from build123d import *

# Parameters (mm, degrees)
EXTRUDE_1_DEPTH     = 4
CUT_EXTRUDE_1_DEPTH = 3
SKETCH_5_R          = 1.25
CUT_EXTRUDE_2_DEPTH = 12.4
SKETCH_13_W         = 36
SKETCH_13_H         = 45
EXTRUDE_2_DEPTH     = 37
SKETCH_14_W         = 13
SKETCH_14_H         = 24
CUT_EXTRUDE_3_DEPTH = 35
SKETCH_15_R         = 1.15
CUT_EXTRUDE_4_DEPTH = 31
SKETCH_16_W         = 10
SKETCH_16_H         = 8
CUT_EXTRUDE_5_DEPTH = 8
SKETCH_17_W         = 36
SKETCH_17_H         = 42.5
CUT_EXTRUDE_6_DEPTH = 18
SKETCH_23_R         = 1.15
CUT_EXTRUDE_7_DEPTH = 5
SKETCH_24_R         = 1.15
CUT_EXTRUDE_8_DEPTH = 5


with BuildPart() as part:
    # 草圖1 → 填料-伸長1 (new body)
    with BuildSketch(Plane.XY):
        with BuildLine():
            Line((7.5, 10), (7.5, 52))
            ThreePointArc((7.5, 52), (0, 59.5), (-7.5, 52))
            Line((-7.5, 52), (-7.5, 10))
            Line((-7.5, 10), (7.5, 10))
        make_face()
    extrude(amount=EXTRUDE_1_DEPTH)

    # 草圖3 → 除料-伸長1 (cut)
    with BuildSketch(Plane.XY):
        with BuildLine():
            ThreePointArc((-2.132795501, 52), (0, 54.132795501), (2.132795501, 52))
            Line((2.132795501, 52), (5, 34.5))
            Line((5, 34.5), (2.114741289, 16.658021353))
            ThreePointArc((2.114741289, 16.658021353), (-0.171540182, 14.864665347), (-2.142213835, 17))
            Line((-2.142213835, 17), (-5, 34.5))
            Line((-5, 34.5), (-2.132795501, 52))
        make_face()
    extrude(amount=CUT_EXTRUDE_1_DEPTH, mode=Mode.SUBTRACT)

    # 草圖5 → 除料-伸長2 (cut)
    with BuildSketch(Plane.XY):
        with Locations((0, 34.5)):
            Circle(SKETCH_5_R)
    extrude(amount=CUT_EXTRUDE_2_DEPTH, mode=Mode.SUBTRACT)

    # 草圖13 → 填料-伸長2 (add)
    with BuildSketch(Plane.XY.offset(4)):
        with Locations((0, -12.5)):
            Rectangle(SKETCH_13_W, SKETCH_13_H)
    extrude(amount=-EXTRUDE_2_DEPTH)

    # 草圖14 → 除料-伸長3 (cut)
    with BuildSketch(Plane(origin=(0, 0, 4), x_dir=(-1, 0, 0), z_dir=(0, 0, -1))):
        with Locations((0, -17)):
            Rectangle(SKETCH_14_W, SKETCH_14_H)
    extrude(amount=CUT_EXTRUDE_3_DEPTH, mode=Mode.SUBTRACT)

    # 草圖15 → 除料-伸長4 (cut)
    with BuildSketch(Plane.XY.offset(4)):
        with Locations((0, -1.85)):
            Circle(SKETCH_15_R)
        with Locations((0, -32.65)):
            Circle(SKETCH_15_R)
    extrude(amount=-CUT_EXTRUDE_4_DEPTH, mode=Mode.SUBTRACT)

    # 草圖16 → 除料-伸長5 (cut)
    with BuildSketch(Plane(origin=(0, -35, 0), x_dir=(-1, 0, 0), z_dir=(0, -1, 0))):
        with Locations((0, 25)):
            Rectangle(SKETCH_16_W, SKETCH_16_H)
    extrude(amount=-CUT_EXTRUDE_5_DEPTH, mode=Mode.SUBTRACT)

    # 草圖17 → 除料-伸長6 (cut)
    with BuildSketch(Plane.XY.offset(4)):
        with Locations((0, -13.75)):
            Rectangle(SKETCH_17_W, SKETCH_17_H)
    extrude(amount=-CUT_EXTRUDE_6_DEPTH, mode=Mode.SUBTRACT)

    # 草圖23 → 除料-伸長7 (cut)
    with BuildSketch(Plane.ZY.offset(18)):
        with Locations((-30, 7)):
            Circle(SKETCH_23_R)
        with Locations((-30, -32)):
            Circle(SKETCH_23_R)
    extrude(amount=-CUT_EXTRUDE_7_DEPTH, mode=Mode.SUBTRACT)

    # 草圖24 → 除料-伸長8 (cut)
    with BuildSketch(Plane(origin=(18, 0, 0), x_dir=(0, 0, -1), z_dir=(1, 0, 0))):
        with Locations((30, 7)):
            Circle(SKETCH_24_R)
        with Locations((30, -32)):
            Circle(SKETCH_24_R)
    extrude(amount=-CUT_EXTRUDE_8_DEPTH, mode=Mode.SUBTRACT)


solid = part.part
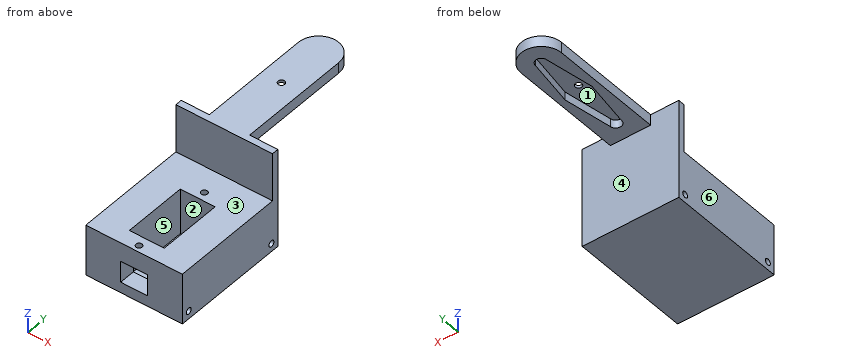
Can you work these out from the model? Positions are in its coordinate system, mm. Face numbers are marked on the shaded views. A direction names the side the tool comes from. Coordinates: 2 decimals unless noted, no trailing zeros. Loops run counter-clockwise (first coordinate to the right, second up) from the corner with the lowest first, then second, coordinate; pieces in that order, holes last. Notation, with made-up numbers: (40, -5) - (58, -5) arc R27 cw to (58, 11) - close; hole circle Ø3 at (72.25, 33). An arc over 180 degrees is marked (long way). Answer as a JSON object with one key per item and string values. Group by question number.
Item 1: On a 3-axis mill with a long thin cutter (end or side, diameter ignored), from which of +Z, -Z, +X, -X, +Y, -Y can I reach the whole of each face in a straight line? I mean the marked faces 1, 2 and 3. Say none if no direction works.
Item 2: If we section it at B-B (z = -25.5): List the corners of the cut face in (x, y) for me, plus the area to 3 significant figures.
Item 3: For pin 1 (5 mm diameter, centred on x = 12.5, z = -1.5, fed in from -Y); pin 2 (5 mm diameter, centred on x = 9, z = -18, fed in from +Y); pin 3 (8 mm diameter, centred on x = 9, y = 13, fed in from -Z); pin 4 (2.5 mm diameter, centred on x = 0, y = -2.5, fed in from +Z), each with a flat end and sliding along its axis, tell me the tip position at first contact or that it passes through.
Item 4: If we section it at D-D (z = -15): List the corners of the cut face in (x, y) for me, plus the area to 3 significant figures.
Item 5: If I drill on L1, parallel to Y at x = -16.05, z = -30; L2, parallel to X at y = -12.5, z = -28; L3, parallel to Y at x = 0, z = -16.25, over which ranges is the centre line in solid material (lowest first)? Write a range as from..to.
Item 6: If we mould it in two halves opening along Y, with no side actions, what happens to the marked faces 4, 5 and 6? For each: released by +Y, released by -Y, zero draft, split by the parting line, or undercut.
Item 7: If we section it at C-C (y = -21): List the corners of the cut face in (x, z) for me.
Item 8: If we section it at A-A (x = 0): State how many separate pieces and enclosed holes the cut face has, plus the area to 3 significant figures.
Returned:
{
 "1": {"face 1": "-Z", "face 2": "+Z", "face 3": "+Z, +X, -X, -Y"},
 "2": {"outline": "(-18, -35) - (-5, -35) - (-5, -29) - (-6.5, -29) - (-6.5, -5) - (6.5, -5) - (6.5, -29) - (5, -29) - (5, -35) - (18, -35) - (18, 10) - (-18, 10) - close; hole circle Ø2.3 at (0, -1.85)", "area": "1,240 mm²"},
 "3": {"pin 1": "stops at y = 7.5", "pin 2": "stops at y = 10", "pin 3": "stops at z = -33", "pin 4": "stops at z = -14"},
 "4": {"outline": "(-18, -35) - (18, -35) - (18, 10) - (-18, 10) - close; hole (-6.5, -29) - (6.5, -29) - (6.5, -5) - (-6.5, -5) - close; hole circle Ø2.3 at (0, -32.65); hole circle Ø2.3 at (0, -1.85)", "area": "1,300 mm²"},
 "5": {"L1": "y = -35..-33.15, -30.85..5.85, 8.15..10", "L2": "x = -18..-6.5, 6.5..18", "L3": "y = -35..-33.8, -31.5..-29, -5..-3, -0.7..10"},
 "6": {"face 4": "released by +Y", "face 5": "undercut", "face 6": "zero draft"},
 "7": {"outline": "(-18, -33) - (18, -33) - (18, -14) - (6.5, -14) - (6.5, -31) - (-6.5, -31) - (-6.5, -14) - (-18, -14) - close"},
 "8": {"separate pieces": "4", "enclosed holes": "0", "area": "476 mm²"}
}
